Work out the finished part from the listing and answer in its coordinate system (mm). Face numbers are marked on the shaded views. A direction names the side the tool comes from. Round coordinates to 2 decimals unless told otherwise and drop trailing zeros. Write each loop counter-clockwise with the first axis right and the second up, starting at its lowest first coordinate (ties: lowest second). Pieces come first, ordered by that corner, then holes. Notation, with made-up numbers: (-27.75, 78) - (-13.75, 78) arc R14 ccw to (-13.75, 99) - close; hole circle Ø8 at (33.5, -34). An arc over 180 degrees is marked (long way). Answer as a JSON object with one key per item and string values.
```python
from build123d import *

# Parameters (mm, degrees)
SKETCH1_R               = 11
BOSS_EXTRUDE1_DEPTH     = 2
SKETCH2_R               = 5
BOSS_EXTRUDE2_DEPTH     = 8
SKETCH3_R               = 1.585
CUT_EXTRUDE1_DEPTH      = 11
SKETCH4_R               = 1.425
CUT_EXTRUDE2_DEPTH      = 2
CIRPATTERN1_COUNT       = 4
SKETCH5_R               = 1.5
CUT_EXTRUDE3_DEPTH      = 12
CUT_EXTRUDE3_DEPTH_BACK = 12


with BuildPart() as part:
    # Sketch1 → Boss-Extrude1 (new body)
    with BuildSketch(Plane(origin=(0, 0, 0), x_dir=(1, 0, 0), z_dir=(0, 1, 0))):
        Circle(SKETCH1_R)
    extrude(amount=BOSS_EXTRUDE1_DEPTH)

    # Sketch2 → Boss-Extrude2 (add)
    with BuildSketch(Plane(origin=(0, 0, 0), x_dir=(1, 0, 0), z_dir=(0, 1, 0))):
        Circle(SKETCH2_R)
    extrude(amount=-BOSS_EXTRUDE2_DEPTH)

    # Sketch3 → Cut-Extrude1 (cut, through all)
    with BuildSketch(Plane(origin=(0, 2, 0), x_dir=(-1, 0, 0), z_dir=(0, -1, 0))):
        Circle(SKETCH3_R)
    extrude(amount=CUT_EXTRUDE1_DEPTH, mode=Mode.SUBTRACT)

    # Sketch4 → Cut-Extrude2 (cut)
    with BuildSketch(Plane(origin=(0, 2, 0), x_dir=(1, 0, 0), z_dir=(0, 1, 0))):
        with Locations((0, 8)):
            Circle(SKETCH4_R)
    cut_extrude2 = extrude(amount=-CUT_EXTRUDE2_DEPTH, mode=Mode.SUBTRACT)

    # CirPattern1: Cut-Extrude2 ×4 about axis
    cirpattern1_axis = Axis((0, 0, 0), (0, 1, 0))
    for i in range(1, CIRPATTERN1_COUNT):
        add(cut_extrude2.rotate(cirpattern1_axis, i * 360 / CIRPATTERN1_COUNT), mode=Mode.SUBTRACT)

    # Sketch5 → Cut-Extrude3 (cut, two sides)
    with BuildSketch(Plane.XY) as cut_extrude3_sk:
        with Locations((0, -4)):
            Circle(SKETCH5_R)
    extrude(amount=CUT_EXTRUDE3_DEPTH, mode=Mode.SUBTRACT)
    extrude(cut_extrude3_sk.sketch, amount=-CUT_EXTRUDE3_DEPTH_BACK, mode=Mode.SUBTRACT)


solid = part.part
```
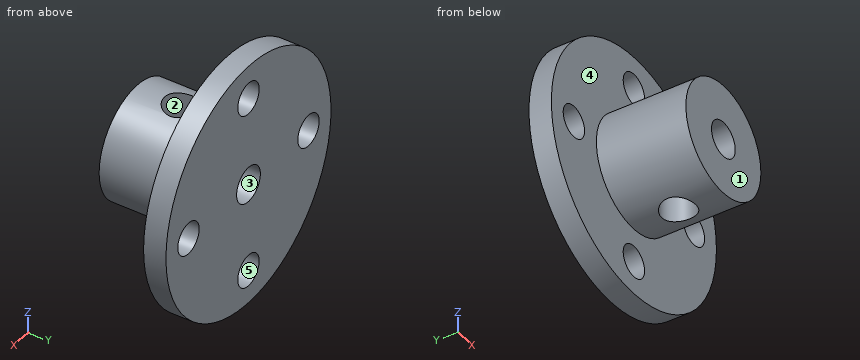
Item 1: A cutting plane is placed at B-B (x = 0). Write down the section's boundary in (y, z) (3 decimals), and give its area (3 significant figures).
Results found:
{"outline": "(-8, -5) - (-5.5, -5) - (-5.5, -1.585) - (-8, -1.585) - close; (-8, 1.585) - (-5.5, 1.585) - (-5.5, 5) - (-8, 5) - close; (-2.5, -5) - (0, -5) - (0, -6.575) - (2, -6.575) - (2, -1.585) - (-2.5, -1.585) - close; (-2.5, 1.585) - (2, 1.585) - (2, 6.575) - (0, 6.575) - (0, 5) - (-2.5, 5) - close; (0, -11) - (2, -11) - (2, -9.425) - (0, -9.425) - close; (0, 9.425) - (2, 9.425) - (2, 11) - (0, 11) - close", "area": "60.4 mm²"}
Item 2: Consider line 1 along X through (y, z) = (1.55, 0) (3 decimals); line 2 along Y through (x, z) = (0, -3.75). Determine where each line is inside the solid, lowest interval first.
Results found:
{"line 1": "-11 to -9.425, -6.575 to -1.585, 1.585 to 6.575, 9.425 to 11", "line 2": "-8 to -5.5, -2.5 to 2"}
Item 3: Each of these flat-tipped pins is pushed along its axis until it touches: P1, Ø5, axis at x = 4.5, y = -5, coming from the -Z side; P2, Ø5, axis at x = 0, y = -4, coming from the -Z side; P3, Ø1.5, axis at x = -1.5, z = -7.5, coming from the -Y side. Where does it stop, or does it pass through?
Results found:
{"P1": "z = -4.58", "P2": "z = -5", "P3": "y = 0"}
Item 4: A cutting plane is placed at A-A (z = 0). Write down the section's boundary in (x, y) (3 decimals).
Results found:
{"outline": "(-11, 0) - (-9.425, 0) - (-9.425, 2) - (-11, 2) - close; (-6.575, 0) - (-5, 0) - (-5, -8) - (-1.585, -8) - (-1.585, 2) - (-6.575, 2) - close; (1.585, -8) - (5, -8) - (5, 0) - (6.575, 0) - (6.575, 2) - (1.585, 2) - close; (9.425, 0) - (11, 0) - (11, 2) - (9.425, 2) - close"}
Item 5: A cutting plane is placed at D-D (x = -8). Write down the section's boundary in (y, z) (3 decimals).
Results found:
{"outline": "(0, -7.55) - (2, -7.55) - (2, -1.425) - (0, -1.425) - close; (0, 1.425) - (2, 1.425) - (2, 7.55) - (0, 7.55) - close"}
Item 6: For the marked faces 4 and 5, determine the directions among +Z, -Z, +X, -X, +Y, -Y from which every point of the face is accessible in a straight line to the end or side of a thin tool.
Results found:
{"face 4": "-Y", "face 5": "+Y, -Y"}
Item 7: A cutting plane is placed at C-C (y = 1.25). Write down the section's boundary in (x, z) (3 decimals).
Results found:
{"outline": "circle Ø22 at (0, 0); hole circle Ø2.85 at (-8, 0); hole circle Ø3.17 at (0, 0); hole circle Ø2.85 at (0, -8); hole circle Ø2.85 at (0, 8); hole circle Ø2.85 at (8, 0)"}
Item 8: Determine the mould class of the marked faces 1, 2 and 3 for opening direction Y: pulls with the +Y half, pulls with the -Y half, needs draft (parallel to the pull), parting line crosses it, or undercut.
Results found:
{"face 1": "pulls with the -Y half", "face 2": "undercut", "face 3": "needs draft"}
